Geometry: final body of the model. Coordinates: model frame, mm. A direction names the side the tool comes from. Give positions to 0.01 mm unless a question says otherwise; leave off trailing zeros. Order: outer loops, then holes, each group sorted by start corner. A loop starts at its lowest first (then second) coordinate and runs counter-clockwise, first axis right, second up. Notation, with made-up numbers: (-40, -31.75) -> (-18, -31.75) arc R22 ccw to (-18, -12.75) -> close; hole circle Ø3 at (46.5, -10.5). An arc over 180 degrees is marked (long way). Answer in a Markdown table with one row per item. Add a question column.
Q1. Cut plane D-D on x = 4. Return the cut outline in (y, z), and give its area (3 significant figures).
Q2. Cut plane A-A on y = 11. Return the cut outline in (x, z).
Q3. Cut plane B-B on z = 15.5. Return the cut outline in (x, y).
Q4. Pull-direction query (Z, two-part tool) for faces 6 (the face through (1.2, 25, -10.6)), 7 (the face through (3.9, 44.5, -3.8)), 8 (the face through (3.9, 4, 13.6)), 9 (the face through (2.37, 1.97, 15.05)); classes: +Z half, -Z half, draft (parallel to the pull), parting line (faces both ways), or undercut.
Q5. Cut plane C-C on x = 7.25. Return the cut outline in (y, z).
Q6. Line query: line 1 along Z through (x, y) = (3.8, 2.3); line 2 along Z through (x, y) = (6.25, 11); line 3 along Y through (x, z) = (4.5, 0). Output: solid intervals per line, ascending. Write a range as from..to.
Q7. Contact query for flat-ended pins moving along their axis: P1, Ø4, axis at x = 2.5, z = -31, coming from the +Y side; P2, Ø1.8, axis at x = 3.8, z = -34.5, coming from the -Y side; P3, Ø4, axis at x = 7, y = 29, coming from the +Z side; P4, Ø1.5, axis at x = 1, z = -4, coming from the -Y side. Output: stop coordinate, or through.
Q8. Set-up query: faces 1 (the face through (4.125, 1.972, -33.036)), 2 (the face through (5.29, 36.92, 1.5)), 3 (the face through (4, 21, -16.5)), 4 (the face through (4, 2, 18.5)), 5 (the face through (4, 22, 8.5)). Return all of +Z, -Z, +X, -X, +Y, -Y with unobstructed straight access to the full face (end or side cutting, diameter ignored); none if empty.
Autodesk Inventor part; units mm, degrees
sketch "Sketch1" plane through (0, 0, 0) normal (1, 0, 0) x (0, 1, 0)
  circle A0 centre (11, 0) radius 6
  circle A1 centre (30.5, -5.5) radius 7.5
  line L0 (0, 29.7) -> (0, -48.7)
  line L1 (-8.9, 0) -> (53.4, 0)
  line L2 (4, 18.5) -> (0, 18.5)
  line L3 (0, -37.5) -> (4, -37.5)
  line L4 (0, 18.5) -> (0, -37.5)
  line L5 (4, 18.5) -> (4, 8.5)
  line L6 (4, -37.5) -> (4, -16.5)
  line L7 (4, -16.5) -> (38.7703, -16.5)
  line L8 (38.7703, 8.5) -> (4, 8.5)
  arc A2 (38.7703, -16.5) -> (38.7703, 8.5) centre (28, -4) ccw
  point P0 (0, 0)
  dimension "d0" = 12
  dimension "d1" = 15
  dimension "d2" = 11
  dimension "d3" = 30.5
  dimension "d4" = 0
  dimension "d5" = 5.5
  dimension "d7" = 56
  dimension "d8" = 4
  dimension "d9" = 4
  dimension "d10" = 0
  dimension "d11" = 0
  dimension "d13" = 11
  dimension "d17" = 16.5
  dimension "d18" = 18.5
  dimension "d19" = 4
  dimension "d20" = 28
  dimension "d21" = 8.5
extrude "Extrusion1" add sketch "Sketch1" along normal blind 8 contours L1 A1 A2 L7 L6 L3 L0 A0 | A0 L1 L0 L2 L5 L8 A2 A1
sketch "Sketch2" plane through (8, 0, 0) normal (1, 0, 0) x (0, 0, -1)
  circle A0 centre (5.5, 30.5) radius 9.5
  line L0 (-18.5, 0) -> (37.5, 0)
  line L1 (0, -8.9) -> (0, 53.4)
  point P0 (0, 0)
  dimension "d24" = 19
  dimension "d25" = 30.5
  dimension "d26" = 5.5
extrude "Extrusion2" cut sketch "Sketch2" against normal blind 5.5
sketch "Sketch3" plane through (0, 0, 0) normal (0, 1, 0) x (-1, 0, 0)
  circle A0 centre (-3.8, 15.5) radius 1.5
  line L0 (-8, 8.5) -> (-8, 18.5)
  line L1 (-9.6, 0) -> (1.6, 0)
  circle A1 centre (-3.8, -34.5) radius 1.5
  line L2 (-8, -37.5) -> (-8, -16.5)
  point P0 (0, 0)
  dimension "d29" = 3
  dimension "d30" = 4.2
  dimension "d31" = 15.5
  dimension "d32" = 3
  dimension "d33" = 4.2
  dimension "d34" = 50
extrude "Extrusion3" cut sketch "Sketch3" along normal blind 4
properties part number "support_arriere_gauche_2"
Completed:
| question | item | result |
|---|---|---|
| 1 | outline | (0, -37.5) -> (4, -37.5) -> (4, -35.99) -> (0, -35.99) -> close; (0, -33.01) -> (4, -33.01) -> (4, -16.5) -> (38.77, -16.5) arc R16.5 ccw to (38.77, 8.5) -> (4, 8.5) -> (4, 14.01) -> (0, 14.01) -> close; (0, 16.99) -> (4, 16.99) -> (4, 18.5) -> (0, 18.5) -> close; hole circle Ø12 at (11, 0); hole circle Ø19 at (30.5, -5.5) |
| 1 | area | 772 mm² |
| 2 | outline | (0, -16.5) -> (8, -16.5) -> (8, -6) -> (0, -6) -> close; (0, 6) -> (8, 6) -> (8, 8.5) -> (0, 8.5) -> close |
| 3 | outline | (0, 0) -> (2.3, 0) -> (2.3, 4) -> (0, 4) -> close; (5.3, 0) -> (8, 0) -> (8, 4) -> (5.3, 4) -> close |
| 4 | face 6 | undercut |
| 4 | face 7 | parting line |
| 4 | face 8 | draft |
| 4 | face 9 | undercut |
| 5 | outline | (0, -37.5) -> (4, -37.5) -> (4, -16.5) -> (38.77, -16.5) arc R16.5 ccw to (38.77, 8.5) -> (4, 8.5) -> (4, 18.5) -> (0, 18.5) -> close; hole circle Ø12 at (11, 0); hole circle Ø19 at (30.5, -5.5) |
| 6 | line 1 | z = -37.5..-36, -33..14, 17..18.5 |
| 6 | line 2 | z = -16.5..-6, 6..8.5 |
| 6 | line 3 | y = 0..5, 17..22.75, 38.25..44.01 |
| 7 | P1 | stops at y = 4 |
| 7 | P2 | passes through |
| 7 | P3 | stops at z = 8.5 |
| 7 | P4 | stops at y = 0 |
| 8 | face 1 | +Y, -Y |
| 8 | face 2 | +X |
| 8 | face 3 | -Z, +X, -X, +Y |
| 8 | face 4 | +Z, +X, -X, +Y, -Y |
| 8 | face 5 | +Z, +X, -X, +Y |
